Design review of the part built by this model. Coordinates are the model's own, in mm. Face numbers are marked on the shaded views. A direction names the side the tool comes from. Give positions to 0.01 mm unless a question says otherwise; leave off trailing zeros. Loops run counter-clockwise (first coordinate to the right, second up) from the corner with the lowest first, then second, coordinate; pieces in that order, holes last.
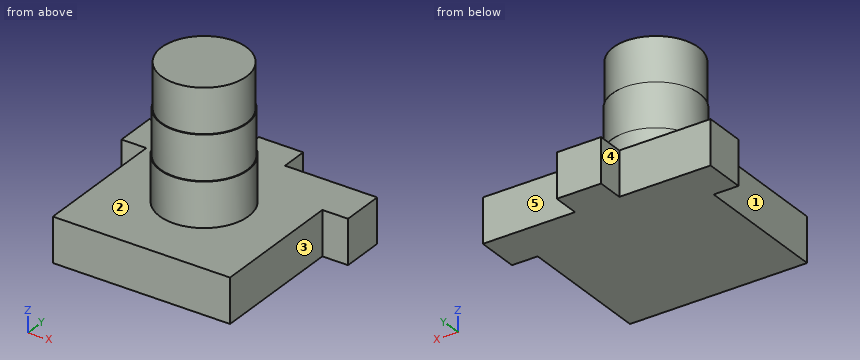
from build123d import *

# Parameters (mm, degrees)
F0_W     = 3.556
F0_H     = 5.842
F0_W_2   = 3.683
F0_H_2   = 6.096
F0_W_3   = 6.35
F0_H_3   = 3.81
F1_DEPTH = 6.35
F2_R     = 6.35
F3_DEPTH = 6.35
F4_R     = 6.223
F5_DEPTH = 6.35
F6_R     = 6.096
F7_DEPTH = 6.35


with BuildPart() as f1:
    # F0 (on Top) → F1 (new body)
    with BuildSketch(Plane.XY):
        Polygon((0, 19.558), (0, 0), (25.4, 0), (25.4, 19.304), (25.4, 25.4), (15.875, 25.4), (9.525, 25.4), (0, 25.4), align=None)
        with Locations((-1.778, 22.479)):
            Rectangle(F0_W, F0_H)
        with Locations((27.2415, 22.352)):
            Rectangle(F0_W_2, F0_H_2)
        with Locations((12.7, 27.305)):
            Rectangle(F0_W_3, F0_H_3)
    extrude(amount=F1_DEPTH)

    # F2 (on face) → F3 (join)
    with BuildSketch(Plane.XY.offset(6.35)):
        with Locations((12.7, 13.10474)):
            Circle(F2_R)
    extrude(amount=F3_DEPTH)

    # F4 (on face) → F5 (join)
    with BuildSketch(Plane.XY.offset(12.7)):
        with Locations((12.7, 13.10474)):
            Circle(F4_R)
    extrude(amount=F5_DEPTH)

    # F6 (on face) → F7 (join)
    with BuildSketch(Plane.XY.offset(19.05)):
        with Locations((12.7, 13.10474)):
            Circle(F6_R)
    extrude(amount=F7_DEPTH)


solid = f1.part
Q1. Take a section at C-C (y = 2.5). Give the boundary of the cut face in (x, z).
Results:
outline: (0, 0) - (25.4, 0) - (25.4, 6.35) - (0, 6.35) - close
Q2. Take a section at B-B (x = 12.7). Give the boundary of the cut face in (y, z), plus the area to 3 significant figures.
Results:
outline: (0, 0) - (29.21, 0) - (29.21, 6.35) - (19.45, 6.35) - (19.45, 12.7) - (19.33, 12.7) - (19.33, 19.05) - (19.2, 19.05) - (19.2, 25.4) - (7.01, 25.4) - (7.01, 19.05) - (6.88, 19.05) - (6.88, 12.7) - (6.75, 12.7) - (6.75, 6.35) - (0, 6.35) - close
area: 423 mm2
Q3. Tool access review of the marked faces 1, 2, 3, 4 and 5: name each direction out of +Z, -Z, +X, -X, +Y, -Y from which nothing blocks a thin tool from reaching the whole face with its end or side.
Results:
face 1: +Z, -Z, -X, -Y
face 2: +Z
face 3: +Z, -Z, +X, -Y
face 4: +Z, -Z, -X, +Y
face 5: +Z, -Z, +X, +Y
Q4. Take a section at D-D (y = 23.25). Give the boundary of the cut face in (x, z).
Results:
outline: (-3.56, 0) - (29.08, 0) - (29.08, 6.35) - (-3.56, 6.35) - close
Q5. Insertion check: pin 1 (3 mm diameter, centred on y = 28, z = 2.5, fed in from +X) (3 decimals); pin 2 (1.9 mm diameter, centred on y = 26.5, z = 4, fed in from -X) (3 decimals); pin 3 (4 mm diameter, centred on x = 6, y = 8, fed in from +Z). Each pin has a flat end and moves straight along its axis. Give the tip position at first contact, or say it passes through.
Results:
pin 1: stops at x = 15.875
pin 2: stops at x = 9.525
pin 3: stops at z = 6.35
Q6. Take a section at A-A (z = 5.5). Give the boundary of the cut face in (x, y) (3 decimals).
Results:
outline: (-3.556, 19.558) - (0, 19.558) - (0, 0) - (25.4, 0) - (25.4, 19.304) - (29.083, 19.304) - (29.083, 25.4) - (15.875, 25.4) - (15.875, 29.21) - (9.525, 29.21) - (9.525, 25.4) - (-3.556, 25.4) - close
Q7. Wall thickness on line 1 (Y direction, x = 24, z = 6.25); line 2 (Z direction, x = 0.5, y = 10.5); line 3 (Y direction, x = 17, z = 13): over which ranges is each line inside the solid? List them lowest first.
Results:
line 1: y = 0 to 25.4
line 2: z = 0 to 6.35
line 3: y = 8.61 to 17.6
